from build123d import *

# Parameters (mm, degrees)
CYLINDER013_R           = 3.7
CYLINDER013_DEPTH       = 10
CYLINDER013_PITCH_ANGLE = 90
CYLINDER012_R           = 2.2
CYLINDER012_DEPTH       = 50
CYLINDER012_PITCH_ANGLE = 90
CYLINDER011_R           = 6.7
CYLINDER011_DEPTH       = 70
CYLINDER011_ROLL_ANGLE  = 90
CYLINDER010_R           = 4.2
CYLINDER010_DEPTH       = 70
CYLINDER010_ROLL_ANGLE  = 90
BOX005009006_W          = 17
BOX005009006_H          = 4
BOX005009006_DEPTH      = 4
BOX005009006_ROLL_ANGLE = 45
BOX005007_W             = 47.5
BOX005007_H             = 21
BOX005007_DEPTH         = 54
FILLET002_R             = 10
CHAMFER007_SIZE         = 10


with BuildPart() as cylinder012:
    # Cylinder013 → Cylinder013 (new body)
    with BuildSketch(Plane.XY):
        Circle(CYLINDER013_R)
    extrude(amount=CYLINDER013_DEPTH)


with BuildPart() as cylinder012_1:
    # Cylinder013 pitch: moved
    add(cylinder012.part.rotate(Axis((0, 0, 0), (0, 1, 0)), CYLINDER013_PITCH_ANGLE))


with BuildPart() as cylinder012_2:
    # Cylinder013 placement: moved
    add(cylinder012_1.part.moved(Location((-15, 496, 2))))


with BuildPart() as cylinder:
    # Cylinder012 → Cylinder012 (new body)
    with BuildSketch(Plane.XY):
        Circle(CYLINDER012_R)
    extrude(amount=CYLINDER012_DEPTH)


with BuildPart() as cylinder_1:
    # Cylinder012 pitch: moved
    add(cylinder.part.rotate(Axis((0, 0, 0), (0, 1, 0)), CYLINDER012_PITCH_ANGLE))


with BuildPart() as cylinder_2:
    # Cylinder012 placement: moved
    add(cylinder_1.part.moved(Location((-12, 496, 2))))


with BuildPart() as m4_screw001:
    # Fusion006 base: copy of Cylinder
    add(cylinder_2.part)

    # Fusion006: union Cylinder012
    add(cylinder012_2.part)


with BuildPart() as m4_screw001_1:
    # Fusion006 placement: moved
    add(m4_screw001.part.moved(Location((0, 0, -9))))


with BuildPart() as fusion007:
    # Fusion005 base: copy of Cylinder
    add(cylinder_2.part)

    # Fusion005: union Cylinder012
    add(cylinder012_2.part)


with BuildPart() as fusion007_1:
    # Fusion005 placement: moved
    add(fusion007.part.moved(Location((0, 0, -30))))

    # Fusion007: union M4-screw001
    add(m4_screw001_1.part)


with BuildPart() as cylinder011:
    # Cylinder011 → Cylinder011 (new body)
    with BuildSketch(Plane.XY):
        Circle(CYLINDER011_R)
    extrude(amount=CYLINDER011_DEPTH)


with BuildPart() as cylinder011_1:
    # Cylinder011 roll: moved
    add(cylinder011.part.rotate(Axis((0, 0, 0), (1, 0, 0)), CYLINDER011_ROLL_ANGLE))


with BuildPart() as cylinder011_2:
    # Cylinder011 placement: moved
    add(cylinder011_1.part.moved(Location((7.75, 569, 2))))


with BuildPart() as cylinder010:
    # Cylinder010 → Cylinder010 (new body)
    with BuildSketch(Plane.XY):
        Circle(CYLINDER010_R)
    extrude(amount=CYLINDER010_DEPTH)


with BuildPart() as cylinder010_1:
    # Cylinder010 roll: moved
    add(cylinder010.part.rotate(Axis((0, 0, 0), (1, 0, 0)), CYLINDER010_ROLL_ANGLE))


with BuildPart() as cylinder010_2:
    # Cylinder010 placement: moved
    add(cylinder010_1.part.moved(Location((7.75, 531, 2))))


with BuildPart() as bracket_blank003:
    # Box005009006 → Box005009006 (new body)
    with BuildSketch(Plane.XY):
        with Locations((8.5, 2)):
            Rectangle(BOX005009006_W, BOX005009006_H)
    extrude(amount=BOX005009006_DEPTH)


with BuildPart() as bracket_blank003_1:
    # Box005009006 roll: moved
    add(bracket_blank003.part.rotate(Axis((0, 0, 0), (1, 0, 0)), BOX005009006_ROLL_ANGLE))


with BuildPart() as bracket_blank003_2:
    # Box005009006 placement: moved
    add(bracket_blank003_1.part.moved(Location((-9, 486.586, -0.8))))


with BuildPart() as bracket:
    # Box005007 → Box005007 (new body)
    with BuildSketch(Plane(origin=(-9, 486, -35), x_dir=(1, 0, 0), z_dir=(0, 0, 1))):
        with Locations((23.75, 10.5)):
            Rectangle(BOX005007_W, BOX005007_H)
    extrude(amount=BOX005007_DEPTH)

    # Fusion004: union bracket-blank003
    add(bracket_blank003_2.part)

    # Cut012: cut Cylinder010
    add(cylinder010_2.part, mode=Mode.SUBTRACT)

    # Cut013: cut Cylinder011
    add(cylinder011_2.part, mode=Mode.SUBTRACT)

    # Cut014: cut Fusion007
    add(fusion007_1.part, mode=Mode.SUBTRACT)

    # Fillet002
    fillet002_edges = [bracket.edges().sort_by_distance(p)[0] for p in [
        (-9, 496.5, 19),
    ]]
    fillet(fillet002_edges, radius=FILLET002_R)

    # Chamfer007
    chamfer007_edges = [bracket.edges().sort_by_distance(p)[0] for p in [
        (38.5, 496.5, 19),
    ]]
    chamfer(chamfer007_edges, length=CHAMFER007_SIZE)


solid = bracket.part
Source: CAD feature listing. Evaluate the final solid. Frame: model axes, mm. A direction names the side the tool comes from. Coordinates: 2 decimals unless noted, no trailing zeros. Loops run counter-clockwise (first coordinate to the right, second up) from the corner with the lowest first, then second, coordinate; pieces in that order, holes last. Notation, with made-up numbers: (11, -25.5) - (37, -25.5) arc R20 ccw to (37, -12.5) - close; hole circle Ø9 at (24, 41.25). An arc over 180 degrees is marked (long way). One line per item, written item: value. Start each with the question number.
1. Section A-A (y = 491). Return the cut outline in (x, z), and give its area (3 significant figures).
2. Mould query, pull axis Z, two halves, no side actions, for faces 1 (the flat face through (-5, 494, -30)), 2 (the flat face through (33.6, 496.4, 13.9)), 3 (the flat face through (-2.502, 484.894, 0.892)), 4 (the flat face through (14, 486, -8)). Classes: pulls with the +Z half, pulls with the -Z half, needs draft (parallel to the pull), parting line crosses it, or undercut.
3. Set-up query: faces 5 (the flat face through (38, 496, -28)), 6 (the cylindrical face through (3.554, 491.485, 2.185)). Return all of +Z, -Z, +X, -X, +Y, -Y with unobstructed straight access to the full face (end or side cutting, diameter ignored); none if empty.
4. Section D-D (z = -28). Return the cut outline in (x, y).
5. Ray query, L1, parallel to Y at x = 18, z = -28; L2, parallel to Z at x = 7.75, y = 487; L3, parallel to Y at x = 25.5, z = -20.5. Return the intervals inside material, ascending.
6. Contact query for flat-ended pins moving along their axis: P1, Ø5.5, axis at y = 496, z = -7, coming from the -X side; P2, Ø8, axis at x = 7.75, z = 2, coming from the -Y side; P3, Ø3, axis at x = 12, z = 2, coming from the -Y side; P4, Ø3.5, axis at y = 496, z = -28, coming from the -X side. Output: stop coordinate, or through.
7. Section C-C (x = 21.5). Return the cut outline in (y, z), and give its area (3 significant figures).
8. Section B-B (x = 7.75). Return the cut outline in (y, z), and give its area (3 significant figures).
Verdict:
1. outline: (-9, -35) - (38.5, -35) - (38.5, 9) - (28.5, 19) - (1, 19) arc R10 ccw to (-9, 9) - close; hole circle Ø8.4 at (7.75, 2)
1. area: 2,440 mm2
2. face 1: undercut
2. face 2: pulls with the +Z half
2. face 3: pulls with the -Z half
2. face 4: needs draft
3. face 5: -X
3. face 6: +Y, -Y
4. outline: (-9, 486) - (38.5, 486) - (38.5, 507) - (-9, 507) - (-9, 499.7) - (-5, 499.7) - (-5, 498.2) - (38, 498.2) - (38, 493.8) - (-5, 493.8) - (-5, 492.3) - (-9, 492.3) - close
5. L1: y = 486 to 493.8, 498.2 to 507
5. L2: z = -35 to -2.2, 6.2 to 19
5. L3: y = 486 to 507
6. P1: stops at x = -5
6. P2: passes through
6. P3: stops at y = 486
6. P4: stops at x = 38
7. outline: (486, -35) - (507, -35) - (507, 19) - (486, 19) - close; hole circle Ø4.4 at (496, -28); hole circle Ø4.4 at (496, -7)
7. area: 1,100 mm2
8. outline: (486, -35) - (507, -35) - (507, -4.7) - (499, -4.7) - (499, -2.2) - (486, -2.2) - close; (486, 6.2) - (499, 6.2) - (499, 8.7) - (507, 8.7) - (507, 19) - (486, 19) - close; hole circle Ø4.4 at (496, -28); hole circle Ø4.4 at (496, -7)
8. area: 887 mm2
